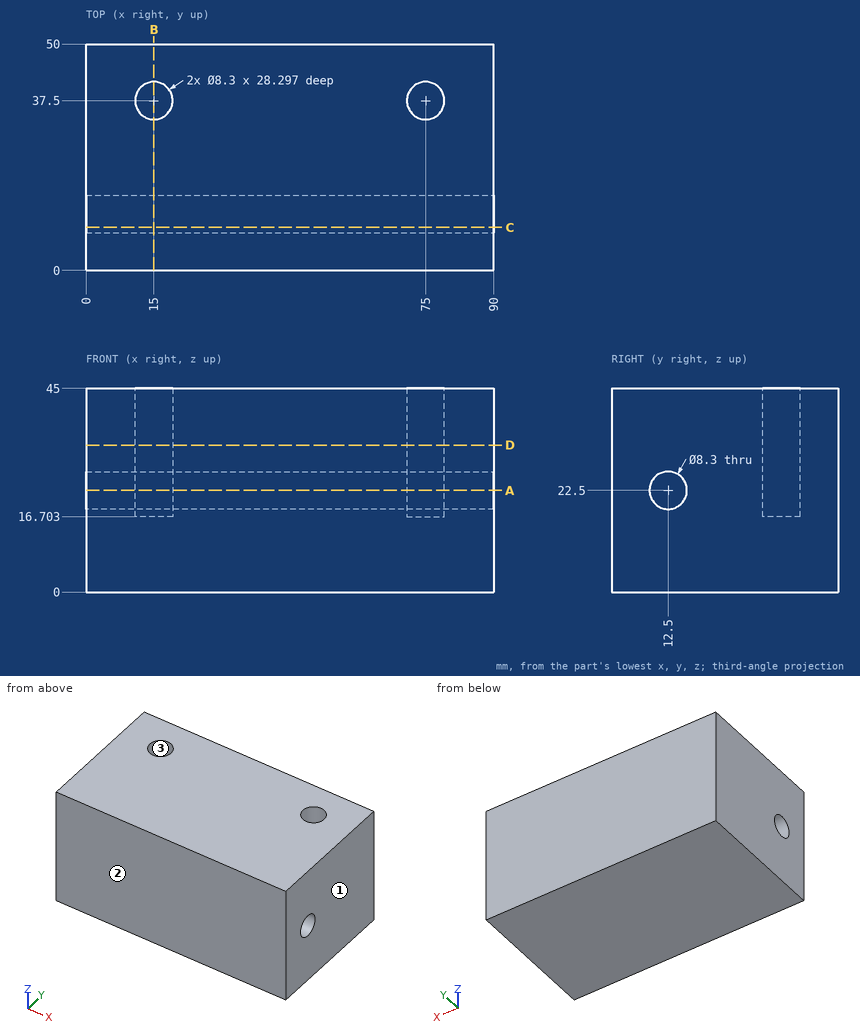
Part print with two shaded views. Sizes in mm from the minimum x, y, z corner. Round coordinates to 2 decimals unless told otherwise and drop trailing zeros. Order: outer loops, then holes, each group sorted by start corner. A loop starts at its lowest first (then second) coordinate and runs counter-clockwise, first axis right, second up. Notation, with made-up numbers: M 4,21.5 L 43,21.5 A12 ccw 43,30.5 Z; hole C 48.5,70 d6. An arc over 180 degrees is marked long. Answer in a Markdown table with one row per item. Add a question column.
Q1. Mould opens along X. For the marked faces 1, 2 and 3 say: +X half, -X half, draft (parallel to the pull), parting line (faces both ways), or undercut.
Q2. Cut at B-B on x = 15. Give the cut face in (y, z).
Q3. Cut at A-A on z = 22.5. Give the cut face in (x, y).
Q4. Wall check: L1, parallel to Y at x = 21, z = 22.5; L2, parallel to Y at x = 75, z = 31.5; L3, parallel to X at y = 37, z = 26. Give the ranges that are in metal, low to high. Write a range as from..to.
Q5. Cut at D-D on z = 32.5. Give the cut face in (x, y), and give its area (3 significant figures).
Q6. Cut at C-C on y = 9.5. Give the cut face in (x, z).
Q7. Pin check, flat tips, straight feed: pin 1 (3 mm diameter, centred on x = 48.5, z = 20.5, fed in from -Y); pin 2 (2.5 mm diameter, centred on x = 73.5, y = 36.5, fed in from +Z). Stop position of each tip, or through.
Established:
| question | item | result |
|---|---|---|
| 1 | face 1 | +X half |
| 1 | face 2 | draft |
| 1 | face 3 | undercut |
| 2 | outline | M 0,0 L 50,0 L 50,45 L 41.65,45 L 41.65,16.7 L 33.35,16.7 L 33.35,45 L 0,45 Z; hole C 12.5,22.5 d8.3 |
| 3 | outline | M 0,0 L 90,0 L 90,8.35 L 0,8.35 Z; M 0,16.65 L 90,16.65 L 90,50 L 0,50 Z; hole C 15,37.5 d8.3; hole C 75,37.5 d8.3 |
| 4 | L1 | y = 0..8.35, 16.65..50 |
| 4 | L2 | y = 0..33.35, 41.65..50 |
| 4 | L3 | x = 0..10.88, 19.12..70.88, 79.12..90 |
| 5 | outline | M 0,0 L 90,0 L 90,50 L 0,50 Z; hole C 15,37.5 d8.3; hole C 75,37.5 d8.3 |
| 5 | area | 4,390 mm2 |
| 6 | outline | M 0,0 L 90,0 L 90,19.63 L 0,19.63 Z; M 0,25.37 L 90,25.37 L 90,45 L 0,45 Z |
| 7 | pin 1 | stops at y = 0 |
| 7 | pin 2 | stops at z = 16.7 |
